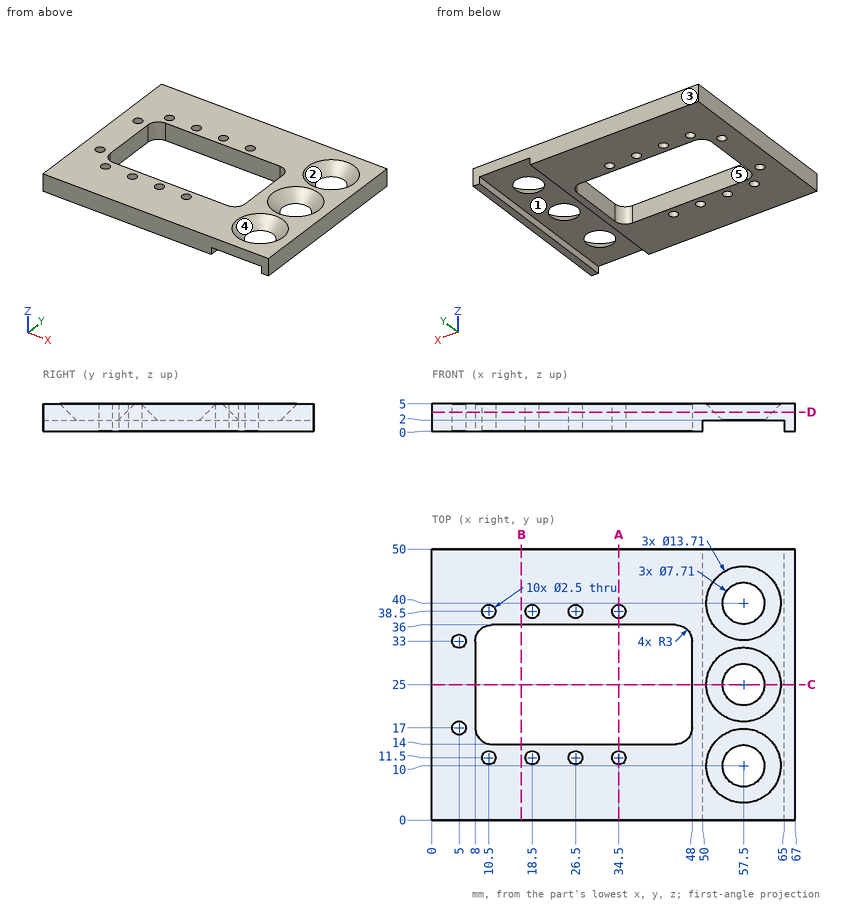
Design review of the part shown in the three views and the two pictorial views. Dimensions are in mm from the part's minimum x, y and z. A direction names the side the tool comes from. Give positions to 0.01 mm unless a question says otherwise; leave off trailing zeros. Write each loop counter-clockwise with the first axis right and the second up, starting at its lowest first coordinate (ties: lowest second). Pieces come first, ordered by that corner, then holes.
(1) Add section A-A (x = 34.5). Give the boundary of the cut face in (y, z), and give its area (3 significant figures).
Checked values:
outline: (0, 0) - (10.25, 0) - (10.25, 5) - (0, 5) - close; (12.75, 0) - (14, 0) - (14, 5) - (12.75, 5) - close; (36, 0) - (37.25, 0) - (37.25, 5) - (36, 5) - close; (39.75, 0) - (50, 0) - (50, 5) - (39.75, 5) - close
area: 115 mm2
(2) Mouldability with a two-part tool opening along Y and no side actions: class the marked faces 1, 2 and 3 as +Y half, -Y half, draft (parallel to the pull), parting line (faces both ways), or undercut.
Checked values:
face 1: draft
face 2: undercut
face 3: +Y half
(3) Add section C-C (y = 25). Give the boundary of the cut face in (x, z) (3 decimals), and give its area (3 significant figures).
Checked values:
outline: (0, 0) - (8, 0) - (8, 5) - (0, 5) - close; (48, 0) - (50, 0) - (50, 2) - (53.645, 2) - (50.645, 5) - (48, 5) - close; (61.355, 2) - (65, 2) - (65, 0) - (67, 0) - (67, 5) - (64.355, 5) - close
area: 72.9 mm2
(4) Add section D-D (z = 3.5). Give the number of separate pieces and of enclosed holes in the cut face, and give its area (3 significant figures).
Checked values:
separate pieces: 1
enclosed holes: 14
area: 2,160 mm2
(5) Clearance check with a flat-ended pin moving along its axis: pin 1 Ø8 at (x, y) = (24, 30.5) entering from -Z. State where the tip first meets the part, or that it passes through.
Checked values:
pin 1: passes through
(6) Add section B-B (x = 16.5). Give the boundary of the cut face in (y, z).
Checked values:
outline: (0, 0) - (14, 0) - (14, 5) - (0, 5) - close; (36, 0) - (50, 0) - (50, 5) - (36, 5) - close
(7) Wall thickness on line 1 along X through (y, z) = (27, 1.75); line 2 along Y through (x, z) = (34.5, 3.05); line 3 along X through (y, z) = (20, 3.9): over which ranges is each line inside the solid? List them lowest first.
Checked values:
line 1: x = 0 to 8, 48 to 50, 65 to 67
line 2: y = 0 to 10.25, 12.75 to 14, 36 to 37.25, 39.75 to 50
line 3: x = 0 to 8, 48 to 54.65, 60.35 to 67
(8) Tool access review of the marked faces 4 and 5: name each direction out of +Z, -Z, +X, -X, +Y, -Y from which nothing blocks a thin tool from reaching the whole face with its end or side.
Checked values:
face 4: +Z
face 5: +Z, -Z
